Check sheet for the drawn part. Datum: minimum x, y, z corner. Units: mm. A direction names the side the tool comes from. Round coordinates to 2 decimals unless told otherwise and drop trailing zeros. Write each loop counter-clockwise with the first axis right and the second up, starting at its lowest first coordinate (ties: lowest second). Pieces come first, ordered by that corner, then holes. Notation, with made-up numbers: (37, 9) - (53, 9) arc R18 cw to (53, 38) - close; hole circle Ø9 at (54.25, 81). An arc over 180 degrees is marked (long way). Answer as a JSON object with one key per item and string values.
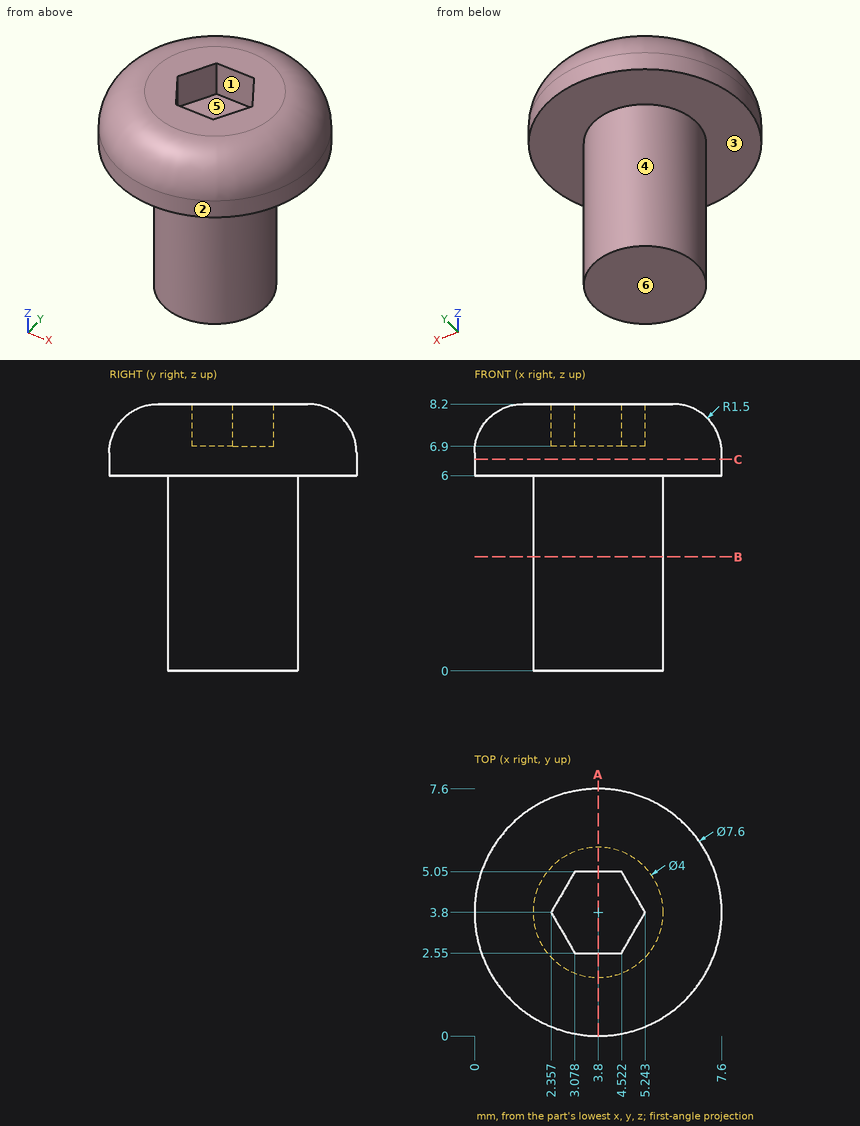
1. Go/stop test with flat-tipped pins: pin 1 (1 mm diameter, centred on x = 4, z = 7.5, fed in from -Y); pin 2 (3 mm diameter, centred on x = 3, y = 4.5, fed in from +Z); pin 3 (4 mm diameter, centred on x = 2.5, z = 3.5, fed in from -Y); pin 4 (1.4 mm diameter, centred on x = 4, z = 8, fed in from +Y). Record where each tip stops, or that it passes through.
Completed:
{"pin 1": "stops at y = 0.03", "pin 2": "stops at z = 8.2", "pin 3": "stops at y = 1.8", "pin 4": "stops at y = 7.47"}
2. Cross-section at A-A (x = 3.8). Record the boundary of the cut face in (y, z), plus the area to 3 significant figures.
Completed:
{"outline": "(0, 6) - (1.8, 6) - (1.8, 0) - (5.8, 0) - (5.8, 6) - (7.6, 6) - (7.6, 6.7) arc R1.5 ccw to (6.1, 8.2) - (5.05, 8.2) - (5.05, 6.9) - (2.55, 6.9) - (2.55, 8.2) - (1.5, 8.2) arc R1.5 ccw to (0, 6.7) - close", "area": "36.5 mm^2"}
3. Access from +Z, -Z, +X, -X, +Y, -Y to the whole of each face (thin tool, end or side, straight path). Record for the marked faces 4, 5 and 6.
Completed:
{"face 4": "-Z", "face 5": "+Z", "face 6": "-Z, +X, -X, +Y, -Y"}
4. Cross-section at C-C (z = 6.5). Record the boundary of the cut face in (x, y).
Completed:
{"outline": "circle Ø7.6 at (3.8, 3.8)"}
5. Mould release check, pull along Y, two halves, no side actions. Record for the marked faces 1, 2 and 3: released by +Y, released by -Y, zero draft, split by the parting line, or undercut.
Completed:
{"face 1": "undercut", "face 2": "split by the parting line", "face 3": "zero draft"}
6. Material ranges on probe 1 along X at (y, z) = (3.75, 0.5); probe 2 along Z at (x, y) = (3.75, 3); probe 3 along Z at (x, y) = (1.5, 3.25), recorded low to high. Write a range as from..to.
Completed:
{"probe 1": "x = 1.8..5.8", "probe 2": "z = 0..6.9", "probe 3": "z = 6..8.2"}
7. Cross-section at B-B (z = 3.5). Record the boundary of the cut face in (x, y).
Completed:
{"outline": "circle Ø4 at (3.8, 3.8)"}
